```python
from build123d import *

# Parameters (mm, degrees)
SKETCH1_R                  = 2.2479
SKETCH1_R_2                = 1.725
BASE_FLANGE1_DEPTH         = 1.5748
SKETCHED_START             = 68.796428764
SKETCHED_BEND1_OUTLINE_W   = 50.8
SKETCHED_BEND1_OUTLINE_H   = 1.5748
SKETCHED_BEND1_DEPTH       = 48.903571236
SKETCHED_START_2           = 65.888620508
SKETCHED_BEND1_2_OUTLINE_W = 50.8
SKETCHED_BEND1_2_OUTLINE_H = 49.865020508
SKETCHED_BEND1_2_OUTLINE_R = 1.725
SKETCHED_BEND1_2_DEPTH     = 3.2512
SKETCHED_START_3           = -26
SKETCHED_BEND1_3_DEPTH     = 52


with BuildPart() as part:
    # Base-Flange1: sheet metal written as solids
    # Sketch1 → Base-Flange1 (new body)
    with BuildSketch(Plane.XY):
        Polygon((12.7, 25.4), (117.7, 25.4), (117.7, -25.4), (12.7, -25.4), (-12.7, -25.4), (-12.7, 25.4), align=None)
        with Locations((-6.35, 19.05)):
            Circle(SKETCH1_R, mode=Mode.SUBTRACT)
        with Locations((6.35, 19.05)):
            Circle(SKETCH1_R, mode=Mode.SUBTRACT)
        with Locations((6.35, 6.35)):
            Circle(SKETCH1_R, mode=Mode.SUBTRACT)
        with Locations((6.35, -6.35)):
            Circle(SKETCH1_R, mode=Mode.SUBTRACT)
        with Locations((6.35, -19.05)):
            Circle(SKETCH1_R, mode=Mode.SUBTRACT)
        with Locations((-6.35, 6.35)):
            Circle(SKETCH1_R, mode=Mode.SUBTRACT)
        with Locations((-6.35, -6.35)):
            Circle(SKETCH1_R, mode=Mode.SUBTRACT)
        with Locations((-6.35, -19.05)):
            Circle(SKETCH1_R, mode=Mode.SUBTRACT)
        with Locations((97.7, 15)):
            Circle(SKETCH1_R_2, mode=Mode.SUBTRACT)
        with Locations((112.7, 15)):
            Circle(SKETCH1_R_2, mode=Mode.SUBTRACT)
        with Locations((112.7, -15)):
            Circle(SKETCH1_R_2, mode=Mode.SUBTRACT)
        with Locations((97.7, -15)):
            Circle(SKETCH1_R_2, mode=Mode.SUBTRACT)
    extrude(amount=-BASE_FLANGE1_DEPTH)

    # Sketched Bend1: read off the stored shape, not the designer's step
    # Sketched Bend1 outline → Sketched Bend1 (cut)
    with BuildSketch(Plane.YZ.offset(SKETCHED_START)):
        with Locations((0, -0.7874)):
            Rectangle(SKETCHED_BEND1_OUTLINE_W, SKETCHED_BEND1_OUTLINE_H)
    extrude(amount=SKETCHED_BEND1_DEPTH, mode=Mode.SUBTRACT)

    # Sketched Bend1 2 outline → Sketched Bend1 2 (add)
    with BuildSketch(Plane.YZ.offset(SKETCHED_START_2)):
        with Locations((0, 24.932510254)):
            Rectangle(SKETCHED_BEND1_2_OUTLINE_W, SKETCHED_BEND1_2_OUTLINE_H)
        with Locations((-15, 29.865020508)):
            Circle(SKETCHED_BEND1_2_OUTLINE_R, mode=Mode.SUBTRACT)
        with Locations((-15, 44.865020508)):
            Circle(SKETCHED_BEND1_2_OUTLINE_R, mode=Mode.SUBTRACT)
        with Locations((15, 29.865020508)):
            Circle(SKETCHED_BEND1_2_OUTLINE_R, mode=Mode.SUBTRACT)
        with Locations((15, 44.865020508)):
            Circle(SKETCHED_BEND1_2_OUTLINE_R, mode=Mode.SUBTRACT)
    extrude(amount=SKETCHED_BEND1_2_DEPTH)

    # Sketched Bend1 3 outline → Sketched Bend1 3 (cut)
    with BuildSketch(Plane(origin=(0, 0, 0), x_dir=(1, 0, 0), z_dir=(0, 1, 0)).offset(SKETCHED_START_3)):
        with BuildLine():
            ThreePointArc((65.888620508, 1.5748), (68.187566075, 0.622545567), (69.139820508, -1.6764))
            Line((69.139820508, -1.6764), (69.139820508, 0))
            Line((69.139820508, 0), (68.796428764, 0))
            Line((68.796428764, 0), (68.796428764, 1.5748))
            Line((68.796428764, 1.5748), (65.888620508, 1.5748))
        make_face()
        with BuildLine():
            Line((67.565020508, -49.865020508), (67.565020508, -1.6764))
            ThreePointArc((67.565020508, -1.6764), (67.074014316, -0.491006192), (65.888620508, 0))
            Line((65.888620508, 0), (65.888620508, -49.865020508))
            Line((65.888620508, -49.865020508), (67.565020508, -49.865020508))
        make_face()
    extrude(amount=SKETCHED_BEND1_3_DEPTH, mode=Mode.SUBTRACT)


solid = part.part
```
Read the model definition and answer for the solid it produces. Units are mm, in the model's axes. A direction names the side the tool comes from. Give positions to 0.01 mm unless a question says otherwise; leave off trailing zeros. Write each loop counter-clockwise with the first axis right and the second up, starting at its lowest first coordinate (ties: lowest second). Pieces come first, ordered by that corner, then holes. Notation, with made-up numbers: (-25, -15.5) -> (24, -15.5) arc R24 ccw to (24, 23.5) -> close; hole circle Ø9 at (-7, 63). An arc over 180 degrees is marked (long way). Answer in a Markdown table with one row per item.
1) A tool of negligible diameter and unlimited length cuts with its end or side. For faces 1 (the flat face through (67.565, 0, 26)), 2 (the cylindrical face through (-4.2, 7, -0.8)), from which of +Z, -Z, +X, -X, +Y, -Y can it reach the whole face along a straight path? Write none if from no direction.
Results list:
| item | result |
|---|---|
| face 1 | +Z, -X, +Y, -Y |
| face 2 | +Z, -Z |
2) Each of these flat-tipped pins is pushed along its axis until it touches: pin 1 Ø7 at (x, y) = (-6.35, 19.05) entering from +Z; pin 2 Ø3 at (y, z) = (-15, 44.87) entering from -X; pin 3 Ø8 at (y, z) = (10.5, 16) entering from -X (3 decimals). Where does it stop, or does it pass through?
Results list:
| item | result |
|---|---|
| pin 1 | z = 0 |
| pin 2 | through |
| pin 3 | x = 67.565 |
3) Section C-C on y = -15 is taken. Give the vertices of the cut face in (x, z).
Results list:
| item | result |
|---|---|
| outline | (-12.7, -1.57) -> (65.89, -1.57) arc R3.25 ccw to (69.14, 1.68) -> (69.14, 28.14) -> (67.57, 28.14) -> (67.57, 1.68) arc R1.68 cw to (65.89, 0) -> (-12.7, 0) -> close; (67.57, 31.59) -> (69.14, 31.59) -> (69.14, 43.14) -> (67.57, 43.14) -> close; (67.57, 46.59) -> (69.14, 46.59) -> (69.14, 49.87) -> (67.57, 49.87) -> close |
4) Section A-A on y = 19.05 is taken. Give the vertices of the cut face in (x, z), plus the area to 3 significant figures.
Results list:
| item | result |
|---|---|
| outline | (-12.7, -1.57) -> (-8.6, -1.57) -> (-8.6, 0) -> (-12.7, 0) -> close; (-4.1, -1.57) -> (4.1, -1.57) -> (4.1, 0) -> (-4.1, 0) -> close; (8.6, -1.57) -> (65.89, -1.57) arc R3.25 ccw to (69.14, 1.68) -> (69.14, 49.87) -> (67.57, 49.87) -> (67.57, 1.68) arc R1.68 cw to (65.89, 0) -> (8.6, 0) -> close |
| area | 192 mm^2 |
5) Straight lines are drawn through the part: line 1 (Y direction, x = 6.35, z = -0.5); line 2 (X direction, y = -13.5, z = 40); line 3 (Z direction, x = 58, y = 14.5). For each, find the intervals that lie inside material, in ascending order. Write a range as [from, to].
Results list:
| item | result |
|---|---|
| line 1 | [-25.4, -21.3], [-16.8, -8.6], [-4.1, 4.1], [8.6, 16.8], [21.3, 25.4] |
| line 2 | [67.57, 69.14] |
| line 3 | [-1.57, 0] |
6) Section B-B on x = -6.35 is taken. Give the vertices of the cut face in (y, z), plus the area to 3 significant figures.
Results list:
| item | result |
|---|---|
| outline | (-25.4, -1.57) -> (-21.3, -1.57) -> (-21.3, 0) -> (-25.4, 0) -> close; (-16.8, -1.57) -> (-8.6, -1.57) -> (-8.6, 0) -> (-16.8, 0) -> close; (-4.1, -1.57) -> (4.1, -1.57) -> (4.1, 0) -> (-4.1, 0) -> close; (8.6, -1.57) -> (16.8, -1.57) -> (16.8, 0) -> (8.6, 0) -> close; (21.3, -1.57) -> (25.4, -1.57) -> (25.4, 0) -> (21.3, 0) -> close |
| area | 51.7 mm^2 |
7) Determine the mould class of faces 3 (the flat face through (28, -25.4, -1)), 4 (the flat face through (69.14, 0, 26)), 5 (the cylindrical face through (8.426, -7.211, -0.776)) for opening direction X: released by +X, released by -X, zero draft, split by the parting line, or undercut.
Results list:
| item | result |
|---|---|
| face 3 | zero draft |
| face 4 | released by +X |
| face 5 | undercut |
8) Section D-D on x = 42.5 is taken. Give the vertices of the cut face in (y, z), plus the area to 3 significant figures.
Results list:
| item | result |
|---|---|
| outline | (-25.4, -1.57) -> (25.4, -1.57) -> (25.4, 0) -> (-25.4, 0) -> close |
| area | 80.0 mm^2 |
